Autodesk Inventor part; units mm, degrees
ref_plane "YZ Plane" through (0, 0, 0) normal (1, 0, 0) x (0, 1, 0)
ref_plane "XZ Plane" through (0, 0, 0) normal (0, 1, 0) x (-1, 0, 0)
ref_plane "XY Plane" through (0, 0, 0) normal (0, 0, 1) x (1, 0, 0)
sketch "Sketch1" plane through (0, 0, 0) normal (1, 0, 0) x (0, 1, 0)
  line L0 (-66.294, 254) -> (66.294, 254)
  line L1 (66.294, 254) -> (66.294, -254)
  line L2 (66.294, -254) -> (-66.294, -254)
  line L3 (-66.294, -254) -> (-66.294, 254)
  line L4 (-66.294, 254) -> (66.294, -254) construction
  line L5 (66.294, 254) -> (-66.294, -254) construction
  point P0 (0, 0)
  dimension "d0" = 508
  dimension "d1" = 132.588
extrude "pdu nmt right side panel" add sketch "Sketch1" along normal blind 3.175
sketch "snap psu" plane through (0, 0, 0) normal (-1, 0, 0) x (0, 0, 1)
  line L0 (-21.209, -49.5046) -> (-21.209, 49.5046) construction
  line L1 (-21.209, 49.5046) -> (190.5, 49.5046) construction
  line L2 (190.5, 49.5046) -> (190.5, -49.5046) construction
  line L3 (190.5, -49.5046) -> (-21.209, -49.5046) construction
  line L4 (179.5018, -49.5046) -> (179.5018, 49.5046) construction
  line L5 (-254, 66.294) -> (254, 66.294)
  line L6 (254, -66.294) -> (254, 66.294)
  line L7 (159.512, 11.5062) -> (159.512, -19.2811) construction
  line L8 (-8.509, 39.497) -> (-8.509, -39.497) construction
  line L9 (124.5108, 0) -> (186.1095, 0) construction
  point P0 (0, 0)
  point P1 (159.512, -39.497)
  dimension "d19" = 10.0076
  dimension "d20" = 30.988
  dimension "d21" = 99.0092
  dimension "d22" = 12.7
  dimension "d23" = 10.9982
  dimension "d24" = 16.7894
  dimension "d25" = 63.5
  dimension "d33" = 10.0076
  dimension "d34" = 89.0016
  dimension "d35" = 30.988
  dimension "d36" = 61.0108
  dimension "d37" = 65.9892
  dimension "d38" = 49.5046
  dimension "d39" = 199.009
  dimension "d40" = 199.009
sketch "Sketch5" plane through (3.175, 0, 0) normal (1, 0, 0) x (0, 0, -1)
  point P0 (0, 0)
  point P1 (8.509, 39.497)
  point P2 (8.509, -39.497)
  point P3 (-124.5108, 0)
  point P4 (-159.512, 11.5062)
  point P5 (-159.512, -39.497)
hole "snap psu holes" at (3.175, 11.5062, 159.512) at (3.175, -39.497, 159.512) at (3.175, 0, 124.5108) at (3.175, 39.497, -8.509) at (3.175, -39.497, -8.509) direction (-1, 0, 0) diameter 3.4036 end through all
sketch "brackets" plane through (3.175, 0, 0) normal (1, 0, 0) x (0, 0, -1)
  line L0 (-254, 66.294) -> (-254, -66.294) construction
  line L1 (-249.428, 54.61) -> (-230.378, 54.61) construction
  line L2 (-230.378, 54.61) -> (-230.378, -54.61) construction
  line L3 (-230.378, -54.61) -> (-249.428, -54.61) construction
  line L4 (-249.428, -54.61) -> (-249.428, 54.61) construction
  line L5 (254, 66.294) -> (-254, 66.294) construction
  line L6 (254, -66.294) -> (254, 66.294) construction
  line L7 (249.428, 54.61) -> (230.378, 54.61) construction
  line L8 (230.378, 54.61) -> (230.378, -54.61) construction
  line L9 (230.378, -54.61) -> (249.428, -54.61) construction
  line L10 (249.428, -54.61) -> (249.428, 54.61) construction
  point P0 (0, 0)
  point P1 (236.3724, 29.21)
  point P2 (236.3724, -29.21)
  point P3 (-236.3724, 29.21)
  point P4 (-236.3724, -29.21)
  dimension "d38" = 49.5046
  dimension "d41" = 11.684
  dimension "d42" = 109.22
  dimension "d43" = 19.05
  dimension "d44" = 11.684
  dimension "d45" = 19.05
  dimension "d46" = 109.22
  dimension "d47" = 25.4
  dimension "d48" = 5.9944
  dimension "d49" = 25.4
  dimension "d50" = 5.9944
  dimension "d51" = 25.4
  dimension "d53" = 25.4
  dimension "d54" = 5.9944
  dimension "d55" = 5.9944
  dimension "d70" = 4.572
  dimension "d71" = 4.572
hole "Hole4" at (3.175, 29.21, -236.3724) at (3.175, -29.21, -236.3724) at (3.175, -29.21, 236.3724) at (3.175, 29.21, 236.3724) direction (-1, 0, 0) diameter 4.2926 end through all countersink diameter 9.398 countersink angle 90
properties part number "nmt_sidepanel_20in"
Check sheet for the modelled part. Datum: model origin and axes. Units: mm. Round coordinates to 2 decimals unless told otherwise and drop trailing zeros. Put each result on its own line as item: value.
(1) Material ranges on line 1 (Z direction, x = 2.6, y = 0); line 2 (Y direction, x = 1.9, z = 126), recorded low to high.
Values found:
line 1: z = -254 to 122.81, 126.21 to 254
line 2: y = -66.29 to -0.82, 0.82 to 66.29
(2) Mould release check, pull along Z, two halves, no side actions. Record for faces 1 (the face through (0.782, -28.517, 234.173)), 2 (the face through (0.78, 29.9, -238.57)), 3 (the face through (3.175, -1, 4)): released by +Z, released by -Z, zero draft, split by the parting line, or undercut.
Values found:
face 1: undercut
face 2: undercut
face 3: zero draft
(3) Go/stop test with flat-tipped pins: pin 1 Ø3 at (y, z) = (39.497, -8.509) entering from +X; pin 2 Ø7 at (y, z) = (29.21, -236.37) entering from +X. Record where each tip stops, or that it passes through.
Values found:
pin 1: passes through
pin 2: stops at x = 1.98
